Can you work these out from the drawing? Everything is in mm from the part's minimum corner. A direction names the side the tool comes from. Coordinates: 2 decimals unless noted, no trailing zeros. Order: outer loops, then holes, each group sorted by start corner. A loop starts at its lowest first (then second) coordinate and runs counter-clockwise, first axis right, second up. Notation, with made-up numbers: (64, 22.5) - (76, 22.5) arc R34 cw to (76, 53.5) - close; hole circle Ø4 at (35.25, 18). An arc over 180 degrees is marked (long way). Use a Markdown table: item, result. Add a question column.
(1) On a 3-axis mill with a long thin cutter (end or side, diameter ignored), from which of +Z, -Z, +X, -X, +Y, -Y can I reach the whole of each face in a straight line? I mean the marked faces 4 and 5. Say none if no direction works.
(2) I want a section at A-A (y = 23.5). List the corners of the cut face in (x, z) for me (1 decimal), and give its area (3 significant figures).
(3) If I drill on L1, parallel to Z at x = 13, y = 61; L2, parallel to Z at x = 67.5, y = 38 (1 decimal); L3, parallel to X at y = 50, z = 70 (1 decimal), over which ranges is the centre line in solid material (lowest first)? Write a range as [from, to].
(4) I want a section at C-C (z = 67). List the corners of the cut face in (x, y) for me (1 decimal).
(5) I want a section at D-D (z = 24.5). List the corners of the cut face in (x, y) for me (1 decimal).
(6) I want a section at B-B (x = 24.5). List the corners of the cut face in (y, z) for me (1 decimal), and give its area (3 significant figures).
(7) We'd pull the mould along X, two halves only. Please class the marked faces 1, 2 and 3: pulls with the +X half, pulls with the -X half, needs draft (parallel to the pull), parting line crosses it, or undercut.
(8) For pin 1 Ø8 at (x, z) = (72, 16) entering from +Y (1 decimal); pin 2 Ø8 at (x, z) = (50.5, 55) entering from -Y; pin 3 Ø5 at (x, y) = (12.5, 44.5) entering from +Z, each with a flat end and sliding along its axis, tell me the tip position at first contact or that it passes through.
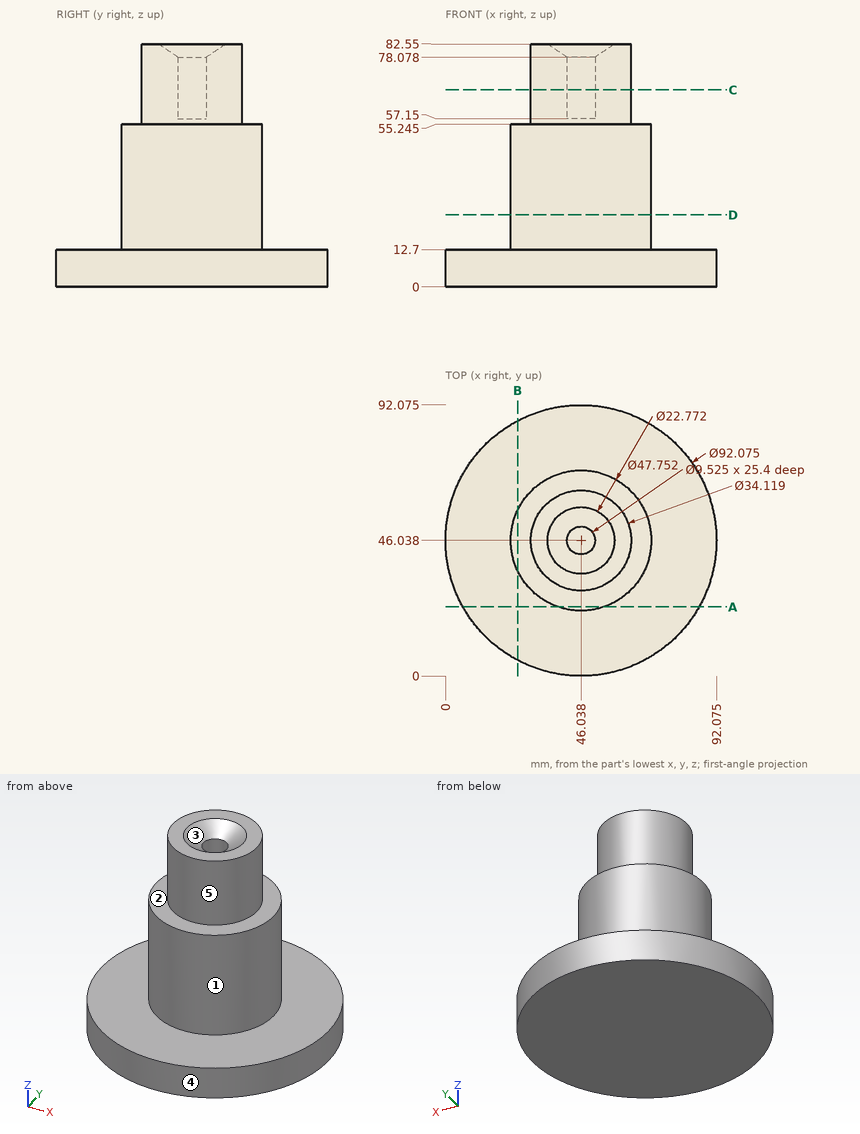
Answers follow:
| question | item | result |
|---|---|---|
| 1 | face 4 | +Z, -Z |
| 1 | face 5 | +Z |
| 2 | outline | (5.9, 0) - (86.2, 0) - (86.2, 12.7) - (53.9, 12.7) - (53.9, 55.2) - (38.2, 55.2) - (38.2, 12.7) - (5.9, 12.7) - close |
| 2 | area | 1,690 mm² |
| 3 | L1 | z = [0, 12.7] |
| 3 | L2 | z = [0, 55.2] |
| 3 | L3 | x = [29.4, 43.4], [48.7, 62.6] |
| 4 | outline | circle Ø34.1 at (46, 46); hole circle Ø9.5 at (46, 46) |
| 5 | outline | circle Ø47.8 at (46, 46) |
| 6 | outline | (5.3, 0) - (86.7, 0) - (86.7, 12.7) - (56.3, 12.7) - (56.3, 55.2) - (35.7, 55.2) - (35.7, 12.7) - (5.3, 12.7) - close |
| 6 | area | 1,910 mm² |
| 7 | face 1 | parting line crosses it |
| 7 | face 2 | needs draft |
| 7 | face 3 | undercut |
| 8 | pin 1 | stops at y = 85.5 |
| 8 | pin 2 | stops at y = 22.17 |
| 8 | pin 3 | stops at z = 12.7 |
